from build123d import *

# Parameters (mm, degrees)
SKETCH1_W           = 39.5
SKETCH1_H           = 39.5
SKETCH1_R           = 6.95
BOSS_EXTRUDE1_DEPTH = 3.65
FILLET1_R           = 5


with BuildPart() as part:
    # Sketch1 → Boss-Extrude1 (new body)
    with BuildSketch(Plane(origin=(0, 0, 0), x_dir=(1, 0, 0), z_dir=(0, 1, 0))):
        Rectangle(SKETCH1_W, SKETCH1_H)
        Circle(SKETCH1_R, mode=Mode.SUBTRACT)
    extrude(amount=BOSS_EXTRUDE1_DEPTH)

    # Fillet1
    fillet1_edges = [part.edges().sort_by_distance(p)[0] for p in [
        (-19.75, 1.825, -19.75),
        (19.75, 1.825, -19.75),
        (19.75, 1.825, 19.75),
        (-19.75, 1.825, 19.75),
    ]]
    fillet(fillet1_edges, radius=FILLET1_R)


solid = part.part
Here's how the part is built. I have some questions about the finished solid (model axes, mm). Coordinates: 2 decimals unless noted, no trailing zeros. Order: outer loops, then holes, each group sorted by start corner. A loop starts at its lowest first (then second) coordinate and runs counter-clockwise, first axis right, second up.
Item 1: If we mould it in two halves opening along X, with no side actions, what happens to faces 1 (the face through (-1.507, 1.799, 6.785)), 2 (the face through (-18.32, 1.85, -18.25)), 3 (the face through (9, 3.65, 0)), 4 (the face through (19.75, 2, 0))? For each: +X half, -X half, draft (parallel to the pull), parting line (faces both ways), or undercut.
Result sheet:
face 1: undercut
face 2: -X half
face 3: draft
face 4: +X half
Item 2: If we section it at C-C on x = 0: List the corners of the cut face in (y, z) for me.
Result sheet:
outline: (0, -19.75) - (3.65, -19.75) - (3.65, -6.95) - (0, -6.95) - close; (0, 6.95) - (3.65, 6.95) - (3.65, 19.75) - (0, 19.75) - close
Item 3: If we section it at B-B on y = 2.7: List the corners of the cut face in (x, z) for me.
Result sheet:
outline: (-19.75, -14.75) arc R5 ccw to (-14.75, -19.75) - (14.75, -19.75) arc R5 ccw to (19.75, -14.75) - (19.75, 14.75) arc R5 ccw to (14.75, 19.75) - (-14.75, 19.75) arc R5 ccw to (-19.75, 14.75) - close; hole circle Ø13.9 at (0, 0)
Item 4: For P1, Ø10, axis at x = -13, z = 8, coming from the -Y side; P2, Ø8.5, axis at x = 0, z = 0, coming from the -Y side, each with a flat end and sliding along its axis, tell me the tip position at first contact or that it passes through.
Result sheet:
P1: stops at y = 0
P2: passes through
Item 5: I need wall thicknesses on line 1 (Z direction, x = 0, y = 2.6); line 2 (X direction, y = 0.45, z = 15). Which ranges of each line are inside material? Lowest first, please.
Result sheet:
line 1: z = -19.75 to -6.95, 6.95 to 19.75
line 2: x = -19.74 to 19.74
Item 6: If we section it at A-A on z = 0: List the corners of the cut face in (x, y) for me.
Result sheet:
outline: (-19.75, 0) - (-6.95, 0) - (-6.95, 3.65) - (-19.75, 3.65) - close; (6.95, 0) - (19.75, 0) - (19.75, 3.65) - (6.95, 3.65) - close
